Part model, mm, in its own coordinate system. A direction names the side the tool comes from. Give positions to 0.01 mm unless a question says otherwise; leave off trailing zeros. Loops run counter-clockwise (first coordinate to the right, second up) from the corner with the lowest first, then second, coordinate; pieces in that order, holes last. Notation, with made-up numbers: M -13.75,9.25 L 23.25,9.25 A9 cw 23.25,26.25 Z; hole C 29.25,-2.75 d5. An arc over 180 degrees is marked long. Answer in a Markdown table with one row per item.
from build123d import *

# Parameters (mm, degrees)
SKETCH1_W           = 50
SKETCH1_H           = 50
SKETCH1_R           = 1.15
BOSS_EXTRUDE1_DEPTH = 2
SKETCH2_W           = 37.6
SKETCH2_H           = 19
BOSS_EXTRUDE2_DEPTH = 10.5
SKETCH3_R           = 3.5
BOSS_EXTRUDE3_DEPTH = 20
SKETCH4_W           = 49
SKETCH4_H           = 49
BOSS_EXTRUDE4_DEPTH = 20


with BuildPart() as part:
    # Sketch1 → Boss-Extrude1 (new body)
    with BuildSketch(Plane(origin=(0, 0, 0), x_dir=(1, 0, 0), z_dir=(0, 1, 0))):
        with Locations((25, 25)):
            Rectangle(SKETCH1_W, SKETCH1_H)
        with Locations(Location((2.5, 3.35, 0), (0, 0, 270))):
            Circle(SKETCH1_R, mode=Mode.SUBTRACT)
        with Locations(Location((47.5, 3.35, 0), (0, 0, 270))):
            Circle(SKETCH1_R, mode=Mode.SUBTRACT)
        with Locations(Location((25, 40.5, 0), (0, 0, 270))):
            Circle(SKETCH1_R, mode=Mode.SUBTRACT)
    extrude(amount=BOSS_EXTRUDE1_DEPTH)

    # Sketch2 → Boss-Extrude2 (add)
    with BuildSketch(Plane(origin=(0, 2, 0), x_dir=(1, 0, 0), z_dir=(0, 1, 0))):
        with Locations((25.6, 10)):
            Rectangle(SKETCH2_W, SKETCH2_H)
    extrude(amount=BOSS_EXTRUDE2_DEPTH)

    # Sketch3 → Boss-Extrude3 (add)
    with BuildSketch(Plane(origin=(0, 2, 0), x_dir=(1, 0, 0), z_dir=(0, 1, 0))):
        with Locations(Location((8, 32, 0), (0, 0, 90))):
            Circle(SKETCH3_R)
    extrude(amount=BOSS_EXTRUDE3_DEPTH)

    # Sketch4 → Boss-Extrude4 (add)
    with BuildSketch(Plane.XZ):
        with Locations((25, -25)):
            Rectangle(SKETCH4_W, SKETCH4_H)
    extrude(amount=BOSS_EXTRUDE4_DEPTH)


solid = part.part
(1) Pin check, flat tips, straight feed: pin 1 Ø3.5 at (x, z) = (47.5, -3.35) entering from +Y; pin 2 Ø21 at (x, z) = (33.5, -8.5) entering from +Y; pin 3 Ø10 at (x, y) = (27.5, -15) entering from -Z. Stop position of each tip, or through.
Recorded:
| item | result |
|---|---|
| pin 1 | stops at y = 2 |
| pin 2 | stops at y = 12.5 |
| pin 3 | stops at z = -49.5 |
(2) Pull direction Z, two halves, no side cores. Call faces 6 (the face through (25, 0, -40)), 7 (the face through (8, 22, -32)), 8 (the face through (25, -10, -49.5)): +Z half, -Z half, draft (parallel to the pull), parting line (faces both ways), or undercut.
Recorded:
| item | result |
|---|---|
| face 6 | undercut |
| face 7 | draft |
| face 8 | -Z half |
(3) Saw through at C-C (y = 13.5). Write the cut outline in (x, z), plus the area to 3 significant figures.
Recorded:
| item | result |
|---|---|
| outline | C 8,-32 d7 |
| area | 38.5 mm^2 |
(4) Saw through at A-A (x = 37.5). Write the cut outline in (y, z), plus the area to 3 significant figures.
Recorded:
| item | result |
|---|---|
| outline | M -20,-49.5 L 0,-49.5 L 0,-50 L 2,-50 L 2,-19.5 L 12.5,-19.5 L 12.5,-0.5 L 2,-0.5 L 2,0 L 0,0 L 0,-0.5 L -20,-0.5 Z |
| area | 1,280 mm^2 |
(5) Which spindle directions (+Z, -Z, +X, -X, +Y, -Y) get a long thin tool onto all of the face, cutting with end or side? Do faces 1 (the face through (0.5, -10, -25)), 2 (the face through (49.5, -10, -25)), 3 (the face through (25, 7, -0.5)), 4 (the face through (9.341, 11.86, -35.233)), 5 (the face through (44.4, 7, -10)). Say none if no direction does.
Recorded:
| item | result |
|---|---|
| face 1 | +Z, -Z, -X, -Y |
| face 2 | +Z, -Z, +X, -Y |
| face 3 | +Z, +X, -X, +Y |
| face 4 | +Y |
| face 5 | +Z, -Z, +X, +Y |
(6) Saw through at D-D (z = -26.5). Write the cut outline in (x, y).
Recorded:
| item | result |
|---|---|
| outline | M 0,0 L 0.5,0 L 0.5,-20 L 49.5,-20 L 49.5,0 L 50,0 L 50,2 L 0,2 Z |
(7) Saw through at B-B (z = -10.5). Write the cut outline in (x, y), plus the area to 3 significant figures.
Recorded:
| item | result |
|---|---|
| outline | M 0,0 L 0.5,0 L 0.5,-20 L 49.5,-20 L 49.5,0 L 50,0 L 50,2 L 44.4,2 L 44.4,12.5 L 6.8,12.5 L 6.8,2 L 0,2 Z |
| area | 1,470 mm^2 |
(8) Drill centre lines: line 1 along X through (y, z) = (0.7, -3.35); line 2 along X through (y, z) = (0.6, -40.5); line 3 along Z through (x, y) = (8, 8.5). Where is each one in solid material? Low to high.
Recorded:
| item | result |
|---|---|
| line 1 | x = 0 to 1.35, 3.65 to 46.35, 48.65 to 50 |
| line 2 | x = 0 to 23.85, 26.15 to 50 |
| line 3 | z = -35.5 to -28.5, -19.5 to -0.5 |
